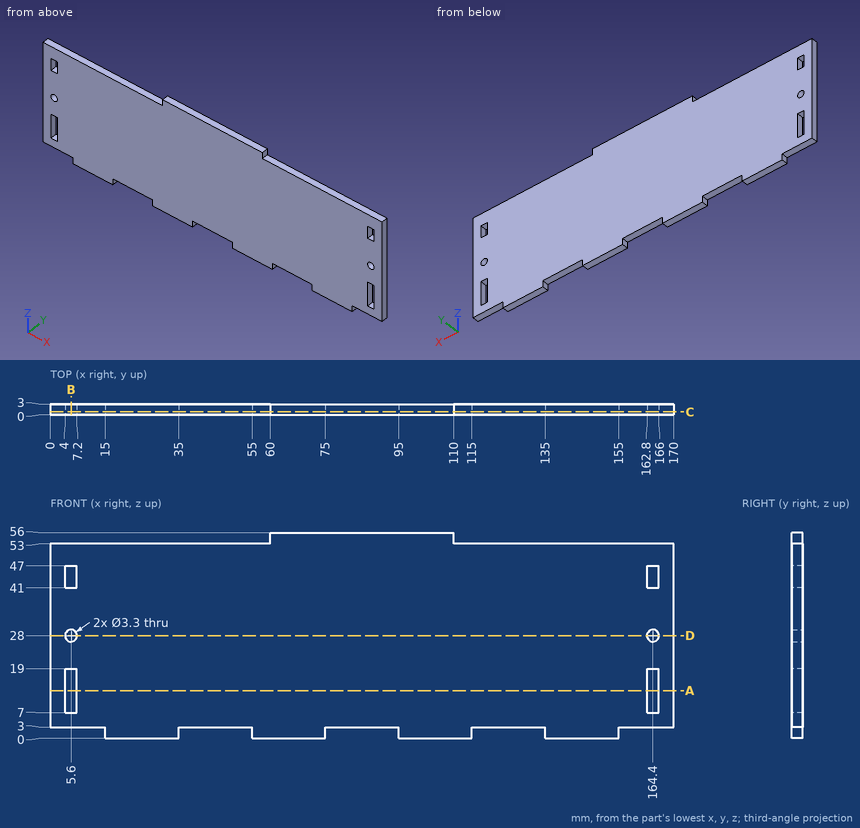
Geometry check sheet. Reference: drawing and pictorial views, mm from the part's lowest x, y, z. Give positions to 0.01 mm unless a question says otherwise; leave off trailing zeros. Order: outer loops, then holes, each group sorted by start corner. A loop starts at its lowest first (then second) coordinate and runs counter-clockwise, first axis right, second up. Notation, with made-up numbers: M -37,66.5 L 6,66.5 A31 ccw 6,105.5 Z; hole C 86.25,-21 d1. An arc over 180 degrees is marked long. Answer as a JSON object with one key per item and string values. Group by question number.
1) Cross-section at C-C (y = 0.85). Give the number of separate pieces and of enclosed holes in the cut face, then the cut area to 3 significant figures.
2) Scan lines: line 1 along Z through (x, y) = (5.6, 1.9); line 2 along X through (y, z) = (2.45, 44.5); line 3 along X through (y, z) = (1.85, 2). Record each from-to range of solid material in increasing order. Write a range as [from, to].
3) Cross-section at B-B (x = 5.6). Enter the section's corners in (y, z), then the cut area to 3 significant figures.
4) Cross-section at D-D (z = 28). Enter the section's corners in (x, y).
5) Cross-section at A-A (z = 13). Enter the section's corners in (x, y).
6) Depth check by flat-ended pin: pin 1 Ø1.5 at (y, z) = (2, 1) entering from +X; pin 2 Ø1.5 at (x, y) = (6, 1.5) entering from +Z; pin 3 Ø1.5 at (y, z) = (1.5, 54) entering from -X. Enter the tip coordinate at first touch or a pass-through.
Result sheet:
{
 "1": {"separate pieces": "1", "enclosed holes": "6", "area": "8,760 mm2"},
 "2": {"line 1": "z = [3, 7], [19, 26.35], [29.65, 41], [47, 53]", "line 2": "x = [0, 4], [7.2, 162.8], [166, 170]", "line 3": "x = [15, 35], [55, 75], [95, 115], [135, 155]"},
 "3": {"outline": "M 0,3 L 3,3 L 3,7 L 0,7 Z; M 0,19 L 3,19 L 3,26.35 L 0,26.35 Z; M 0,29.65 L 3,29.65 L 3,41 L 0,41 Z; M 0,47 L 3,47 L 3,53 L 0,53 Z", "area": "86.1 mm2"},
 "4": {"outline": "M 0,0 L 3.95,0 L 3.95,3 L 0,3 Z; M 7.25,0 L 162.75,0 L 162.75,3 L 7.25,3 Z; M 166.05,0 L 170,0 L 170,3 L 166.05,3 Z"},
 "5": {"outline": "M 0,0 L 4,0 L 4,3 L 0,3 Z; M 7.2,0 L 162.8,0 L 162.8,3 L 7.2,3 Z; M 166,0 L 170,0 L 170,3 L 166,3 Z"},
 "6": {"pin 1": "stops at x = 155", "pin 2": "stops at z = 53", "pin 3": "stops at x = 60"}
}
